from build123d import *

# Parameters (mm, degrees)
SKETCH1_W            = 75.2
SKETCH1_H            = 100.2
BOSS_EXTRUDE1_DEPTH  = 1.6
CHAMFER1_SIZE        = 2
SKETCH2_R            = 1.25
CUT_EXTRUDE1_DEPTH   = 2.6
SKETCH3_W            = 8.8
SKETCH3_H            = 58.7
SKETCH3_W_2          = 20.5
SKETCH3_H_2          = 8.9
BOSS_EXTRUDE2_DEPTH  = 9
SKETCH3_3_W          = 20.1
SKETCH3_3_H          = 32
BOSS_EXTRUDE3_DEPTH  = 1.6
SKETCH3_4_W          = 6.3
SKETCH3_4_H          = 21.8
SKETCH3_4_H_2        = 16.2
SKETCH3_4_H_3        = 5.5
BOSS_EXTRUDE4_DEPTH  = 8.6
SKETCH3_5_W          = 10
SKETCH3_5_H          = 9.5
BOSS_EXTRUDE5_DEPTH  = 5.3
SKETCH3_6_W          = 8.9
SKETCH3_6_H          = 14
BOSS_EXTRUDE6_DEPTH  = 10.9
BOSS_EXTRUDE7_DEPTH  = 8
SKETCH5_W            = 43.8
SKETCH5_H            = 2
BOSS_EXTRUDE8_DEPTH  = 3.9
SKETCH7_W            = 42.5
SKETCH7_H            = 24.2
BOSS_EXTRUDE9_DEPTH  = 8.1
SKETCH7_3_W          = 43
SKETCH7_3_H          = 21.4
BOSS_EXTRUDE10_DEPTH = 14
SKETCH8_W            = 20.1
SKETCH8_H            = 24
BOSS_EXTRUDE11_DEPTH = 10
SKETCH9_R            = 1.75
BOSS_EXTRUDE12_DEPTH = 2


with BuildPart() as part:
    # Sketch1 → Boss-Extrude1 (new body)
    with BuildSketch(Plane(origin=(0, 0, 0), x_dir=(1, 0, 0), z_dir=(0, 1, 0))):
        Rectangle(SKETCH1_W, SKETCH1_H)
    extrude(amount=BOSS_EXTRUDE1_DEPTH)

    # Chamfer1
    chamfer1_edges = [part.edges().sort_by_distance(p)[0] for p in [
        (37.6, 0.8, 50.1),
        (-37.6, 0.8, 50.1),
        (-37.6, 0.8, -50.1),
        (37.6, 0.8, -50.1),
    ]]
    chamfer(chamfer1_edges, length=CHAMFER1_SIZE)

    # Sketch2 → Cut-Extrude1 (cut, through all)
    with BuildSketch(Plane(origin=(0, 1.6, 0), x_dir=(1, 0, 0), z_dir=(0, 1, 0))):
        with Locations((-32.2, 44.45)):
            Circle(SKETCH2_R)
        with Locations((-32.2, -44.45)):
            Circle(SKETCH2_R)
        with Locations((31.3, -44.45)):
            Circle(SKETCH2_R)
        with Locations((31.3, 44.45)):
            Circle(SKETCH2_R)
    extrude(amount=-CUT_EXTRUDE1_DEPTH, mode=Mode.SUBTRACT)

    # Sketch3 → Boss-Extrude2 (add)
    with BuildSketch(Plane(origin=(0, 1.6, 0), x_dir=(1, 0, 0), z_dir=(0, 1, 0))):
        with Locations((-28.4, 10.25)):
            Rectangle(SKETCH3_W, SKETCH3_H)
        with Locations((15.55, 45.55)):
            Rectangle(SKETCH3_W_2, SKETCH3_H_2)
    extrude(amount=BOSS_EXTRUDE2_DEPTH)

    # Sketch3<3> → Boss-Extrude3 (add)
    with BuildSketch(Plane(origin=(0, 1.6, 0), x_dir=(1, 0, 0), z_dir=(0, 1, 0))):
        with Locations((-5.75, 33.1)):
            Rectangle(SKETCH3_3_W, SKETCH3_3_H)
    extrude(amount=BOSS_EXTRUDE3_DEPTH)

    # Sketch3<4> → Boss-Extrude4 (add)
    with BuildSketch(Plane(origin=(0, 1.6, 0), x_dir=(1, 0, 0), z_dir=(0, 1, 0))):
        with Locations((34.35, 25.2)):
            Rectangle(SKETCH3_4_W, SKETCH3_4_H)
        with Locations((34.35, 2.7)):
            Rectangle(SKETCH3_4_W, SKETCH3_4_H_2)
        with Locations((34.35, -22.85)):
            Rectangle(SKETCH3_4_W, SKETCH3_4_H_2)
        with Locations((34.35, -35.5)):
            Rectangle(SKETCH3_4_W, SKETCH3_4_H_3)
    extrude(amount=BOSS_EXTRUDE4_DEPTH)

    # Sketch3<5> → Boss-Extrude5 (add)
    with BuildSketch(Plane(origin=(0, 1.6, 0), x_dir=(1, 0, 0), z_dir=(0, 1, 0))):
        with Locations((-9.2, -45.35)):
            Rectangle(SKETCH3_5_W, SKETCH3_5_H)
        with Locations((6, -45.35)):
            Rectangle(SKETCH3_5_W, SKETCH3_5_H)
        with Locations((21.2, -45.35)):
            Rectangle(SKETCH3_5_W, SKETCH3_5_H)
    extrude(amount=BOSS_EXTRUDE5_DEPTH)

    # Sketch3<6> → Boss-Extrude6 (add)
    with BuildSketch(Plane(origin=(0, 1.6, 0), x_dir=(1, 0, 0), z_dir=(0, 1, 0))):
        with Locations((-24.55, -42.6)):
            Rectangle(SKETCH3_6_W, SKETCH3_6_H)
    extrude(amount=BOSS_EXTRUDE6_DEPTH)

    # Sketch4 → Boss-Extrude7 (add)
    with BuildSketch(Plane(origin=(0, 0, -50.1), x_dir=(-1, 0, 0), z_dir=(0, 0, -1))):
        with BuildLine():
            Line((8.5, 3.2), (3, 3.2))
            ThreePointArc((3, 3.2), (1.3, 4.9), (3, 6.6))
            Line((3, 6.6), (8.5, 6.6))
            ThreePointArc((8.5, 6.6), (10.2, 4.9), (8.5, 3.2))
        make_face()
    extrude(amount=-BOSS_EXTRUDE7_DEPTH)

    # Sketch5 → Boss-Extrude8 (add)
    with BuildSketch(Plane(origin=(0, 1.6, 0), x_dir=(1, 0, 0), z_dir=(0, 1, 0))):
        with Locations((6, -46.9)):
            Rectangle(SKETCH5_W, SKETCH5_H)
    extrude(amount=BOSS_EXTRUDE8_DEPTH)

    # Sketch7 → Boss-Extrude9 (add)
    with BuildSketch(Plane(origin=(0, 1.6, 0), x_dir=(1, 0, 0), z_dir=(0, 1, 0))):
        with Locations((1.65, -20)):
            Rectangle(SKETCH7_W, SKETCH7_H)
    extrude(amount=BOSS_EXTRUDE9_DEPTH)

    # Sketch7<3> → Boss-Extrude10 (add)
    with BuildSketch(Plane(origin=(0, 1.6, 0), x_dir=(1, 0, 0), z_dir=(0, 1, 0))):
        with Locations((1.4, 4.8)):
            Rectangle(SKETCH7_3_W, SKETCH7_3_H)
    extrude(amount=BOSS_EXTRUDE10_DEPTH)

    # Sketch8 → Boss-Extrude11 (add)
    with BuildSketch(Plane(origin=(0, 3.2, 0), x_dir=(1, 0, 0), z_dir=(0, 1, 0))):
        with Locations((-5.75, 29.1)):
            Rectangle(SKETCH8_W, SKETCH8_H)
    extrude(amount=BOSS_EXTRUDE11_DEPTH)

    # Sketch9 → Boss-Extrude12 (add)
    with BuildSketch(Plane(origin=(0, 15.6, 0), x_dir=(1, 0, 0), z_dir=(0, 1, 0))):
        with Locations((4.6, 12.6)):
            Circle(SKETCH9_R)
    extrude(amount=BOSS_EXTRUDE12_DEPTH)


solid = part.part
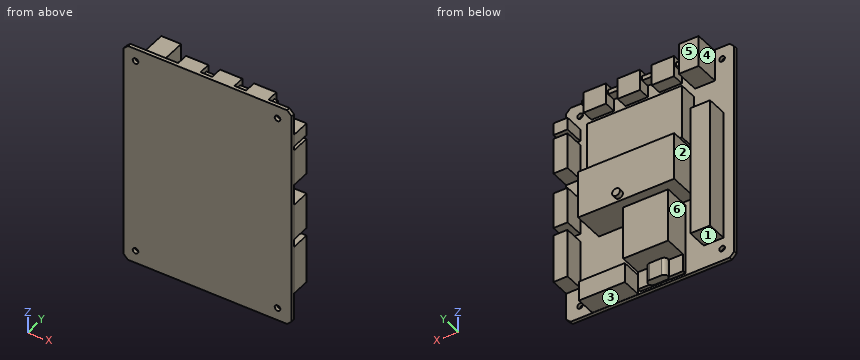
For this review, take the finished solid that the model builds, in its own axes (mm). Face numbers are marked on the shaded views. A direction names the side the tool comes from. Give positions to 0.01 mm unless a question says otherwise; leave off trailing zeros. Order: outer loops, then holes, each group sorted by start corner. A loop starts at its lowest first (then second) coordinate and runs counter-clockwise, first axis right, second up. Notation, with made-up numbers: (-11.5, -28) - (6.5, -28) arc R24 ccw to (6.5, 7) - close; hole circle Ø2 at (43.5, 82.25). An arc over 180 degrees is marked (long way). Answer as a JSON object with one key per item and string values. Group by question number.
Item 1: Take a section at C-C on y = 4.25. Give the number of separate pieces and of enclosed holes in the cut face, and give its area (3 significant figures).
Item 2: Draft analysis for pull direction X (two halves, no side actions). For the marked faces 4, 5 and 6, state which applies: pulls with the +X half, pulls with the -X half, needs draft (parallel to the pull), parting line crosses it, or undercut.
Item 3: Take a section at A-A on z = -35. Give the boundary of the cut face in (x, y).
Item 4: Wall thickness on line 1 along X through (y, z) = (6.75, 1.5); line 2 along Z through (x, y) = (-32.2, 1.25); line 3 along Z through (x, y) = (34, 9.75): over which ranges is each line inside the solid? List them lowest first.
Item 5: Take a section at D-D on x = 9. Give the boundary of the cut face in (y, z), and give its area (3 significant figures).
Item 6: Take a section at B-B on x = -22.5. Give the boundary of the cut face in (y, z), and give its area (3 significant figures).
Item 7: Clearance check with flat-ended pins moving along their axes: pin 1 Ø6 at (y, z) = (9, -37) entering from -X; pin 2 Ø4 at (y, z) = (4.5, 43) entering from -X; pin 3 Ø0.6 at (x, z) = (14, 46.5) entering from +Y. State where each tip first meets the part, or that it passes through.
Item 8: Machinability: for the marked faces 1, 2 and 3, which of the approach directions +Z, -Z, +X, -X, +Y, -Y give a long, thin tool a straight path to every point of the face, cutting with its end or side? Answer none if there is none.
Reported:
{
 "1": {"separate pieces": "12", "enclosed holes": "0", "area": "4,010 mm^2"},
 "2": {"face 4": "pulls with the -X half", "face 5": "needs draft", "face 6": "undercut"},
 "3": {"outline": "(-37.6, 0) - (37.6, 0) - (37.6, 1.6) - (37.5, 1.6) - (37.5, 10.2) - (31.2, 10.2) - (31.2, 1.6) - (4.3, 1.6) - (4.3, 13.2) - (-15.8, 13.2) - (-15.8, 1.6) - (-24, 1.6) - (-24, 10.6) - (-32.8, 10.6) - (-32.8, 1.6) - (-37.6, 1.6) - close"},
 "4": {"line 1": "-32.8 to -24, -20.1 to 22.9, 31.2 to 37.5", "line 2": "-50.1 to -45.7, -43.2 to 43.2, 45.7 to 50.1", "line 3": "-36.1 to -14.3, -10.8 to 5.4, 14.75 to 30.95, 32.75 to 38.25"},
 "5": {"outline": "(0, -50.1) - (1.6, -50.1) - (1.6, -50) - (10.6, -50) - (10.6, -41.1) - (1.6, -41.1) - (1.6, -15.5) - (15.6, -15.5) - (15.6, 5.9) - (1.6, 5.9) - (1.6, 7.9) - (9.7, 7.9) - (9.7, 32.1) - (1.6, 32.1) - (1.6, 40.6) - (6.9, 40.6) - (6.9, 50.1) - (0, 50.1) - close", "area": "786 mm^2"},
 "6": {"outline": "(0, -50.1) - (1.6, -50.1) - (1.6, 35.6) - (12.5, 35.6) - (12.5, 49.6) - (1.6, 49.6) - (1.6, 50.1) - (0, 50.1) - close", "area": "313 mm^2"},
 "7": {"pin 1": "x = -32.8", "pin 2": "x = -29", "pin 3": "y = 5.5"},
 "8": {"face 1": "-Z, -X, +Y", "face 2": "-Z, +Y", "face 3": "-Z, +X, +Y"}
}
